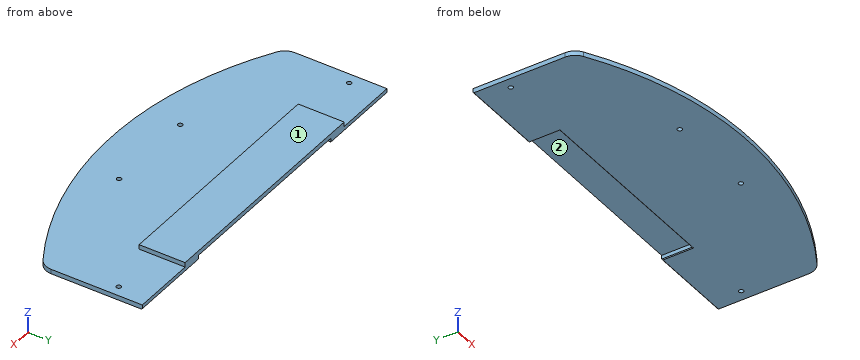
from build123d import *

# Parameters (mm, degrees)
EXTRUDE_1_DEPTH     = 3
SKETCH_2_W          = 156
SKETCH_2_H          = 30
EXTRUDE_2_DEPTH     = 3
SKETCH_3_R          = 1.5
CUT_EXTRUDE_1_DEPTH = 3
SKETCH_4_W          = 130
SKETCH_4_H          = 20
CUT_EXTRUDE_2_DEPTH = 3
FILLET_1_R          = 10
CHAMFER_1_SIZE      = 0.5


with BuildPart() as part:
    # 草图1 → 凸台-拉伸1 (new body)
    with BuildSketch(Plane.XY):
        with BuildLine():
            Line((-120, -25), (120, -25))
            Line((120, -25), (120, -90))
            ThreePointArc((120, -90), (0.09506488, -125.000515914), (-120, -90.658049905))
            Line((-120, -90.658049905), (-120, -25))
        make_face()
    extrude(amount=EXTRUDE_1_DEPTH)

    # 草图2 → 凸台-拉伸2 (add)
    with BuildSketch(Plane.XY.offset(3)):
        with Locations((0, -40)):
            Rectangle(SKETCH_2_W, SKETCH_2_H)
    extrude(amount=EXTRUDE_2_DEPTH)

    # 草图3 → 切除-拉伸1 (cut)
    with BuildSketch(Plane(origin=(0, 0, 0), x_dir=(-1, 0, 0), z_dir=(0, 0, -1))):
        with Locations((30, -100)):
            Circle(SKETCH_3_R)
        with Locations((113, -45)):
            Circle(SKETCH_3_R)
        with Locations(Location((-113, -45, 0), (0, 0, 180))):
            Circle(SKETCH_3_R)
        with Locations(Location((-30, -100, 0), (0, 0, 180))):
            Circle(SKETCH_3_R)
    extrude(amount=-CUT_EXTRUDE_1_DEPTH, mode=Mode.SUBTRACT)

    # 草图4 → 切除-拉伸2 (cut)
    with BuildSketch(Plane(origin=(0, 0, 0), x_dir=(-1, 0, 0), z_dir=(0, 0, -1))):
        with Locations((0, -35)):
            Rectangle(SKETCH_4_W, SKETCH_4_H)
    extrude(amount=-CUT_EXTRUDE_2_DEPTH, mode=Mode.SUBTRACT)

    # 圆角1
    fillet_1_edges = [part.edges().sort_by_distance(p)[0] for p in [
        (120, -90, 1.5),
        (-120, -90.658049905, 1.5),
    ]]
    fillet(fillet_1_edges, radius=FILLET_1_R)

    # 倒角1
    chamfer_1_edges = [part.edges().sort_by_distance(p)[0] for p in [
        (-92.5, -25, 0),
        (92.5, -25, 0),
        (65, -35, 0),
        (0, -45, 0),
        (-65, -35, 0),
    ]]
    chamfer(chamfer_1_edges, length=CHAMFER_1_SIZE)


solid = part.part
Part model, mm, in its own coordinate system. Face numbers are marked on the shaded views. Round coordinates to 2 decimals unless told otherwise and drop trailing zeros. Write each loop counter-clockwise with the first axis right and the second up, starting at its lowest first coordinate (ties: lowest second). Pieces come first, ordered by that corner, then holes. Notation, with made-up numbers: M 63.25,-38 L 82.25,-38 A12 cw 82.25,-15 Z; hole C 49,-38 d9. An arc over 180 degrees is marked long. Return JSON: item names as keys, results as strings. Group by question number.
(1) Saw through at D-D on y = -82. Write the cut outline in (x, z), then the cut area to 3 significant figures.
(2) Two-plate mould, pull along X, no slides. Class the marked faces 1 and 2: +X half, -X half, draft (parallel to the pull), parting line (faces both ways), or undercut.
(3) Saw through at C-C on z = 4.75. Write the cut outline in (x, y).
(4) Saw through at A-A on y = -36.5. Write the cut outline in (x, z), then the cut area to 3 significant figures.
(5) Saw through at B-B on x = -51. Write the cut outline in (y, z).
(6) Drill centre lines: probe 1 along X at (y, z) = (-35, 2); probe 2 along X at (y, z) = (-100, 2.3); probe 3 along Z at (x, y) = (-13.5, -30). Where is each one in solid material? Low to high.
(7) Pin check, flat tips, straight feed: pin 1 Ø2 at (x, z) = (-11.5, 1.5) entering from +Y; pin 2 Ø1.5 at (y, z) = (-35, 5) entering from +X; pin 3 Ø5 at (x, y) = (30, -100) entering from +Z. Stop position of each tip, or through.
Returned:
{
 "1": {"outline": "M -120,0 L 120,0 L 120,3 L -120,3 Z", "area": "720 mm²"},
 "2": {"face 1": "draft", "face 2": "undercut"},
 "3": {"outline": "M -78,-55 L 78,-55 L 78,-25 L -78,-25 Z"},
 "4": {"outline": "M -120,0 L -65.5,0 L -65,0.5 L -65,3 L 65,3 L 65,0.5 L 65.5,0 L 120,0 L 120,3 L 78,3 L 78,6 L -78,6 L -78,3 L -120,3 Z", "area": "798 mm²"},
 "5": {"outline": "M -119.27,0 L -45.5,0 L -45,0.5 L -45,3 L -25,3 L -25,6 L -55,6 L -55,3 L -119.27,3 Z"},
 "6": {"probe 1": "-120 to -65, 65 to 120", "probe 2": "-103.6 to -31.5, -28.5 to 28.5, 31.5 to 102.56", "probe 3": "3 to 6"},
 "7": {"pin 1": "y = -45", "pin 2": "x = 78", "pin 3": "z = 3"}
}
